from build123d import *

# Parameters (mm, degrees)
SKETCH1_W           = 70
SKETCH1_H           = 3
BOSS_EXTRUDE1_DEPTH = 55
SKETCH2_W           = 70
SKETCH2_H           = 2.5
BOSS_EXTRUDE2_DEPTH = 22.8
SKETCH5_R           = 3.5
CUT_EXTRUDE1_DEPTH  = 84.8
SKETCH6_W           = 16
SKETCH6_H           = 11.6
SKETCH6_W_2         = 15
BOSS_EXTRUDE7_DEPTH = 22.8
SKETCH7_R           = 1
CUT_EXTRUDE2_DEPTH  = 8
SKETCH8_R           = 1
CUT_EXTRUDE3_DEPTH  = 8
FILLET1_R           = 5
SKETCH9_W           = 14.084433838
SKETCH9_H           = 7
CUT_EXTRUDE4_DEPTH  = 66


with BuildPart() as part:
    # Sketch1 → Boss-Extrude1 (new body)
    with BuildSketch(Plane.XY):
        Rectangle(SKETCH1_W, SKETCH1_H)
    extrude(amount=BOSS_EXTRUDE1_DEPTH)

    # Sketch2 → Boss-Extrude2 (add)
    with BuildSketch(Plane(origin=(0, 1.5, 0), x_dir=(1, 0, 0), z_dir=(0, 1, 0))):
        with Locations((0, -1.25)):
            Rectangle(SKETCH2_W, SKETCH2_H)
        with Locations((0, -53.75)):
            Rectangle(SKETCH2_W, SKETCH2_H)
    extrude(amount=BOSS_EXTRUDE2_DEPTH)

    # Sketch5 → Cut-Extrude1 (cut)
    with BuildSketch(Plane.XY.offset(55)):
        with Locations((-24, 11.4)):
            Circle(SKETCH5_R)
    extrude(amount=-CUT_EXTRUDE1_DEPTH, mode=Mode.SUBTRACT)

    # Sketch6 → Boss-Extrude7 (add)
    with BuildSketch(Plane(origin=(0, 24.3, 0), x_dir=(1, 0, 0), z_dir=(0, 1, 0))):
        with Locations((-7, -27.5)):
            Rectangle(SKETCH6_W, SKETCH6_H)
        with Locations((27.5, -27.5)):
            Rectangle(SKETCH6_W_2, SKETCH6_H)
    extrude(amount=-BOSS_EXTRUDE7_DEPTH)

    # Sketch7 → Cut-Extrude2 (cut)
    with BuildSketch(Plane(origin=(0, 24.3, 0), x_dir=(1, 0, 0), z_dir=(0, 1, 0))):
        with Locations((-12, -24.7)):
            Circle(SKETCH7_R)
        with Locations((23, -30.3)):
            Circle(SKETCH7_R)
        with Locations((-2, -24.7)):
            Circle(SKETCH7_R)
        with Locations((-2, -30.3)):
            Circle(SKETCH7_R)
        with Locations((-12, -30.3)):
            Circle(SKETCH7_R)
        with Locations((23, -24.7)):
            Circle(SKETCH7_R)
        with Locations((32, -24.7)):
            Circle(SKETCH7_R)
        with Locations((32, -30.3)):
            Circle(SKETCH7_R)
    extrude(amount=-CUT_EXTRUDE2_DEPTH, mode=Mode.SUBTRACT)

    # Sketch8 → Cut-Extrude3 (cut)
    with BuildSketch(Plane(origin=(35, 0, 0), x_dir=(0, 0, -1), z_dir=(1, 0, 0))):
        with Locations((-24.7, 19.3)):
            Circle(SKETCH8_R)
        with Locations((-30.3, 19.3)):
            Circle(SKETCH8_R)
        with Locations((-24.7, 6.5)):
            Circle(SKETCH8_R)
        with Locations((-30.3, 6.5)):
            Circle(SKETCH8_R)
    extrude(amount=-CUT_EXTRUDE3_DEPTH, mode=Mode.SUBTRACT)

    # Fillet1
    fillet1_edges = [part.edges().sort_by_distance(p)[0] for p in [
        (1, 1.5, 27.5),
        (-15, 1.5, 27.5),
        (20, 1.5, 27.5),
    ]]
    fillet(fillet1_edges, radius=FILLET1_R)

    # Sketch9 → Cut-Extrude4 (cut)
    with BuildSketch(Plane.XY.offset(55)):
        with Locations((-31.042216919, 11.4)):
            Rectangle(SKETCH9_W, SKETCH9_H)
    extrude(amount=-CUT_EXTRUDE4_DEPTH, mode=Mode.SUBTRACT)


solid = part.part
The model under review builds one solid part; all positions refer to its coordinate system, in mm. A direction names the side the tool comes from. Round coordinates to 2 decimals unless told otherwise and drop trailing zeros. Order: outer loops, then holes, each group sorted by start corner. A loop starts at its lowest first (then second) coordinate and runs counter-clockwise, first axis right, second up. Notation, with made-up numbers: (2, -1) -> (61, -1) arc R32 cw to (61, 37) -> close; hole circle Ø5 at (-29, -11). An arc over 180 degrees is marked (long way). Use CSV: the item, a comma, the result in double quotes. Start each with the question number.
(1) Wall thickness on probe 1 along X at (y, z) = (20.75, 30.3); probe 2 along Z at (x, y) = (32.8, 19.3); probe 3 along Z at (x, y) = (29, 21.75): over which ranges is each line inside the solid? List them lowest first. Write a range as from..to.
(2) Mouldability with a two-part tool opening along Y and no side actions: class faces 1 (the face through (27, 24.3, 27)), 2 (the face through (29, 19.3, 31.3)), 3 (the face through (-30, 14.9, 54)), 4 (the face through (-15, 16, 28)) as pulls with the +Y half, pulls with the -Y half, needs draft (parallel to the pull), parting line crosses it, or undercut.
(3) Consider section D-D on z = 15.5. Write out the cut boundary in (x, y), and give its area (3 significant figures).
(4) Insertion check: pin 1 (1.2 mm diameter, centred on x = 32, z = 24.7, fed in from +Y); pin 2 (1.2 mm diameter, centred on y = 6.5, z = 24.7, fed in from +X); pin 3 (3.5 mm diameter, centred on y = 15, z = 25.5, fed in from -X). Each pin has a flat end and moves straight along its axis. Give the tip position at first contact, or say it passes through.
(5) Consider section A-A on x = -27.5. Write out the cut boundary in (y, z), and give its area (3 significant figures).
(6) Tool access review of faces 5 (the face through (-7, 13, 33.3)), 6 (the face through (27, 19, 30)), 7 (the face through (18.5, 2.93, 27.42)): name each direction out of +Z, -Z, +X, -X, +Y, -Y from which nothing blocks a thin tool from reaching the whole face with its end or side.
(7) Consider section B-B on y = 11.4. Write out the cut boundary in (x, z), and give its area (3 significant figures).
(8) Consider section C-C on x = -17. Write out the cut boundary in (y, z), and give its area (3 significant figures).
Responses:
1,probe 1,"-15..-13, -11..-3, -1..1, 20..22, 24..31, 33..35"
1,probe 2,"0..2.5, 21.7..23.7, 25.7..29.3, 31.3..33.3, 52.5..55"
1,probe 3,"0..2.5, 21.7..33.3, 52.5..55"
2,face 1,"pulls with the +Y half"
2,face 2,"undercut"
2,face 3,"undercut"
2,face 4,"needs draft"
3,outline,"(-35, -1.5) -> (35, -1.5) -> (35, 1.5) -> (-35, 1.5) -> close"
3,area,"210 mm²"
4,pin 1,"y = 16.3"
4,pin 2,"x = 27"
4,pin 3,"x = -15"
5,outline,"(-1.5, 0) -> (7.9, 0) -> (7.9, 2.5) -> (1.5, 2.5) -> (1.5, 52.5) -> (7.9, 52.5) -> (7.9, 55) -> (-1.5, 55) -> close; (14.9, 0) -> (24.3, 0) -> (24.3, 2.5) -> (14.9, 2.5) -> close; (14.9, 52.5) -> (24.3, 52.5) -> (24.3, 55) -> (14.9, 55) -> close"
5,area,"244 mm²"
6,face 5,"+X, -X, +Y"
6,face 6,"+X"
6,face 7,"+Y"
7,outline,"(-20.5, 0) -> (35, 0) -> (35, 2.5) -> (-20.5, 2.5) -> close; (-20.5, 52.5) -> (35, 52.5) -> (35, 55) -> (-20.5, 55) -> close; (-15, 21.7) -> (1, 21.7) -> (1, 33.3) -> (-15, 33.3) -> close; (20, 21.7) -> (35, 21.7) -> (35, 33.3) -> (20, 33.3) -> close"
7,area,"637 mm²"
8,outline,"(-1.5, 0) -> (24.3, 0) -> (24.3, 2.5) -> (1.5, 2.5) -> (1.5, 21.7) -> (2.5, 21.7) -> (2.5, 33.3) -> (1.5, 33.3) -> (1.5, 52.5) -> (24.3, 52.5) -> (24.3, 55) -> (-1.5, 55) -> close"
8,area,"291 mm²"
